The model under review builds one solid part; all positions refer to its coordinate system, in mm. A direction names the side the tool comes from. Coordinates: 2 decimals unless noted, no trailing zeros. Loops run counter-clockwise (first coordinate to the right, second up) from the corner with the lowest first, then second, coordinate; pieces in that order, holes last. Notation, with made-up numbers: M 43,34 L 75,34 A13 ccw 75,40 Z; hole C 50,51.5 d10. An arc over 180 degrees is marked long. Use CSV: the item, a comma, the result in double quotes. Start each with the question number.
1. Add section B-B, the plane z = 0. Write out the cut boundary in (x, y) (3 decimals), then the cut area to 3 significant figures.
2. Clearance check with a flat-ended pin moving along its axis: P1, Ø2, axis at y = 11.5, z = -0.5, coming from the -X side (3 decimals). State where the tip first meets the part, or that it passes through.
3. For L1, parallel to X at y = 14.5, z = 0 (3 decimals); L2, parallel to X at y = 26, z = -4.5, list the stretches that pass through material, from the lowest coordinate up.
4. Add section A-A, the plane x = 0. Write out the cut boundary in (y, z) (3 decimals).
5. Draft analysis for pull direction X (two halves, no side actions). For faces 4 (the flat face through (3.655, 17, 0)), 5 (the flat face through (-5.38, 17.26, -4.32)), 6 (the flat face through (-10, 17, 6)), 7 (the flat face through (0.1, 35, 2.4)), state which applies: +X half, -X half, draft (parallel to the pull), parting line (faces both ways), or undercut.
6. Tool access review of faces 1 (the flat face through (-6, 17, 10)), 2 (the flat face through (0, 17, 3.655)), 3 (the flat face through (4, 17, 8.5)): name each direction out of +Z, -Z, +X, -X, +Y, -Y from which nothing blocks a thin tool from reaching the whole face with its end or side.
Autodesk Inventor part; units mm, degrees
ref_plane "YZ Plane" through (0, 0, 0) normal (1, 0, 0) x (0, 1, 0)
ref_plane "XZ Plane" through (0, 0, 0) normal (0, 1, 0) x (-1, 0, 0)
ref_plane "XY Plane" through (0, 0, 0) normal (0, 0, 1) x (1, 0, 0)
sketch "Sketch1" plane through (0, 0, 0) normal (0, 1, 0) x (-1, 0, 0)
  line L0 (0, -14) -> (0, 14)
  line L1 (-14, 0) -> (14, 0)
  line L2 (14, 0) -> (-14, 0)
  line L3 (0, -14) -> (0, 14)
  line L4 (2.5943, 3.655) -> (-2.5943, 3.655)
  line L5 (-3.655, 2.5943) -> (-3.655, -2.5943)
  line L6 (-2.5943, -3.655) -> (2.5943, -3.655)
  line L7 (3.655, -2.5943) -> (3.655, 2.5943)
  line L8 (-3.655, 3.655) -> (3.655, -3.655) construction
  line L9 (10, 10) -> (10, 2.63)
  line L10 (10, 2.63) -> (8.5, 2.63)
  line L11 (10, 10) -> (2.63, 10)
  line L12 (2.63, 10) -> (2.63, 8.5)
  line L13 (-10, 10) -> (-2.63, 10)
  line L14 (-2.63, 10) -> (-2.63, 8.5)
  line L15 (-10, 8.5) -> (-10, 10)
  line L16 (-10, 10) -> (-8.5, 10)
  line L17 (-8.5, 2.63) -> (-10, 2.63)
  line L18 (-10, 2.63) -> (-10, 10)
  line L19 (-10, -10) -> (-8.5, -10)
  line L20 (-8.5, -2.63) -> (-10, -2.63)
  line L21 (-10, -2.63) -> (-10, -10)
  line L22 (-10, -10) -> (-2.63, -10)
  line L23 (-2.63, -10) -> (-2.63, -8.5)
  line L24 (-10, -8.5) -> (-10, -10)
  line L25 (10, -10) -> (8.5, -10)
  line L26 (8.5, -2.63) -> (10, -2.63)
  line L27 (10, -2.63) -> (10, -10)
  line L28 (10, -10) -> (2.63, -10)
  line L29 (2.63, -10) -> (2.63, -8.5)
  line L30 (10, -8.5) -> (10, -10)
  circle A0 centre (0, 0) radius 2.095
  line L31 (5.995, -10) -> (2.63, -10)
  line L32 (-2.63, -10) -> (-5.995, -10)
  line L33 (10, -10) -> (2.63, -10)
  line L34 (-2.63, -10) -> (-10, -10)
  line L35 (10, -5.995) -> (10, -2.63)
  line L36 (10, 2.63) -> (10, 5.995)
  line L37 (10, 10) -> (10, 2.63)
  line L38 (10, -2.63) -> (10, -10)
  line L39 (-5.995, 10) -> (-2.63, 10)
  line L40 (2.63, 10) -> (5.995, 10)
  line L41 (-10, 10) -> (-2.63, 10)
  line L42 (2.63, 10) -> (10, 10)
  line L43 (-10, 5.995) -> (-10, 2.63)
  line L44 (-10, -2.63) -> (-10, -5.995)
  line L45 (-10, -10) -> (-10, -2.63)
  line L46 (-10, 2.63) -> (-10, 10)
  line L47 (-2.63, -8.5) -> (-5.995, -8.5)
  line L48 (-8.5, -5.995) -> (-8.5, -2.63)
  line L49 (-8.5, -5.995) -> (-7.0557, -5.995)
  line L50 (-5.995, -8.5) -> (-5.995, -7.0557)
  line L51 (-5.995, 7.0557) -> (-5.995, 8.5)
  line L52 (2.63, 8.5) -> (5.995, 8.5)
  line L53 (8.5, 2.63) -> (8.5, 5.995)
  line L54 (8.5, 5.995) -> (7.0557, 5.995)
  line L55 (5.995, 8.5) -> (5.995, 7.0557)
  line L56 (2.63, -8.5) -> (5.995, -8.5)
  line L57 (9.5607, -8.5) -> (10, -8.5)
  line L58 (8.5, -10) -> (8.5, -9.5607)
  line L59 (8.5, -5.995) -> (8.5, -2.63)
  line L60 (7.0557, -5.995) -> (8.5, -5.995)
  line L61 (5.995, -7.0557) -> (5.995, -8.5)
  line L62 (3.655, 3.655) -> (-0.5303, -0.5303) construction
  line L63 (-1.4814, -1.4814) -> (-3.655, -3.655) construction
  line L64 (-8.5, 10) -> (-8.5, 9.5607)
  line L65 (-8.5, 5.995) -> (-8.5, 2.63)
  line L66 (-2.63, 8.5) -> (-5.995, 8.5)
  line L67 (-9.5607, 8.5) -> (-10, 8.5)
  line L68 (-7.0557, 5.995) -> (-8.5, 5.995)
  line L69 (-3.655, 2.5943) -> (-7.0557, 5.995)
  line L70 (-2.5943, 3.655) -> (-5.995, 7.0557)
  line L71 (5.995, 7.0557) -> (2.5943, 3.655)
  line L72 (7.0557, 5.995) -> (3.655, 2.5943)
  line L73 (7.0557, -5.995) -> (3.655, -2.5943)
  line L74 (5.995, -7.0557) -> (2.5943, -3.655)
  line L75 (-2.5943, -3.655) -> (-5.995, -7.0557)
  line L76 (-3.655, -2.5943) -> (-7.0557, -5.995)
  dimension "d26" = 4.19
  dimension "d0" = 20
  dimension "d1" = 20
  dimension "d2" = 7.31
  dimension "d3" = 7.31
  dimension "d4" = 20
  dimension "d5" = 11.99
  dimension "d6" = 11.99
  dimension "d11" = 7.37
  dimension "d12" = 1.5
  dimension "d13" = 7.37
  dimension "d14" = 1.5
  dimension "d15" = 7.37
  dimension "d16" = 1.5
  dimension "d17" = 7.37
  dimension "d18" = 1.5
  dimension "d19" = 7.37
  dimension "d20" = 7.37
  dimension "d21" = 1.5
  dimension "d22" = 1.5
  dimension "d23" = 7.37
  dimension "d24" = 7.37
  dimension "d25" = 1.5
extrude "Extrusion1" add sketch "Sketch1" along normal blind 35 contours L6 L75 L50 L47 L23 L22 L19 L21 L20 L48 L49 L76 L5 L1 A0 L0 | L0 A0 L1 L7 L73 L60 L59 L26 L27 L25 L28 L29 L56 L61 L74 L6 | L1 L5 L69 L68 L65 L17 L18 L15 L13 L14 L66 L51 L70 L4 L0 A0 | A0 L0 L4 L71 L55 L52 L12 L11 L9 L10 L53 L54 L72 L7 L1
fillet "Fillet1" radius 0.5 20 edges at (10, 17.5, 10) (2.63, 17.5, 10) (-2.63, 17.5, 10) (-2.63, 17.5, 8.5) (10, 17.5, 2.63) (8.5, 17.5, 2.63) (10, 17.5, -2.63) (8.5, 17.5, -2.63) (10, 17.5, -10) (2.63, 17.5, -8.5) (-2.63, 17.5, -10) (-2.63, 17.5, -8.5) (2.63, 17.5, -10) (-10, 17.5, -10) (-8.5, 17.5, -2.63) (-10, 17.5, -2.63) (-8.5, 17.5, 2.63) (-10, 17.5, 2.63) (-10, 17.5, 10) (2.63, 17.5, 8.5)
fillet "Fillet2" radius 0.75 24 edges at (-7.0557, 17.5, 5.995) (-3.655, 17.5, 2.5943) (-8.5, 17.5, -5.995) (-7.0557, 17.5, -5.995) (-5.995, 17.5, -8.5) (3.655, 17.5, -2.5943) (7.0557, 17.5, -5.995) (-2.5943, 17.5, 3.655) (-5.995, 17.5, 7.0557) (3.655, 17.5, 2.5943) (7.0557, 17.5, 5.995) (8.5, 17.5, 5.995) (8.5, 17.5, -5.995) (2.5943, 17.5, 3.655) (5.995, 17.5, 7.0557) (5.995, 17.5, 8.5) (-5.995, 17.5, 8.5) (-8.5, 17.5, 5.995) (2.5943, 17.5, -3.655) (5.995, 17.5, -7.0557) (5.995, 17.5, -8.5) (-5.995, 17.5, -7.0557) (-2.5943, 17.5, -3.655) (-3.655, 17.5, -2.5943)
properties part number "pro35mm"
Computed:
1,outline,"M -3.655,0 L -2.095,0 L -2.095,35 L -3.655,35 Z; M 2.095,0 L 3.655,0 L 3.655,35 L 2.095,35 Z"
1,area,"109 mm^2"
2,P1,"stops at x = -3.655"
3,L1,"x = -3.655 to -2.095, 2.095 to 3.655"
3,L2,"x = -10 to -8.5, -5.56 to -3.44, 3.44 to 5.56, 8.5 to 10"
4,outline,"M 0,-3.655 L 35,-3.655 L 35,-2.095 L 0,-2.095 Z; M 0,2.095 L 35,2.095 L 35,3.655 L 0,3.655 Z"
5,face 4,"+X half"
5,face 5,"undercut"
5,face 6,"-X half"
5,face 7,"draft"
6,face 1,"+Z, +X, -X, +Y, -Y"
6,face 2,"+Z, +Y, -Y"
6,face 3,"+Y, -Y"
